Answer from the drawing. Dimensions are ordinates in mm from the lowest x, y and z of the part. A direction names the side the tool comes from. Coordinates: 2 decimals unless noted, no trailing zeros. Order: outer loops, then holes, each group sorted by start corner. A loop starts at its lowest first (then second) coordinate and runs counter-clockwise, first axis right, second up. Notation, with made-up numbers: (26.5, 61.25) -> (38.5, 61.25) arc R4 cw to (38.5, 68.25) -> close; hole circle Ø2 at (25.25, -2). An arc over 180 degrees is marked (long way). Answer as a JSON object with one key per item and string values. Group by question number.
1) A tool of negligible diameter and unlimited length cuts with its end or side. For the marked faces 1 and 2, from which of +Z, -Z, +X, -X, +Y, -Y can it reach the whole face along a straight path? Write none if from no direction.
2) Consider L1, parallel to Z at x = 33, y = 19.5; L2, parallel to X at y = 28, z = 31 (1 decimal); L3, parallel to X at y = 31.5, z = 26 (1 decimal). Determine where each line is inside the solid, lowest interval first.
3) Given pin 1 (4 mm diameter, centred on y = 19, z = 30, fed in from +X) (1 decimal); pin 2 (8 mm diameter, centred on y = 27.5, z = 22, fed in from -X); pin 3 (12 mm diameter, centred on y = 21, z = 25, fed in from +X), each flat-ended and moving along its own axis, determine where each tip first touches the part or whether it passes through.
4) Section B-B on x = 36 is taken. Determine the outline of the cut face in (y, z) (1 decimal), and give its area (3 significant figures).
5) Section C-C on z = 29 is taken. Determine the outline of the cut face in (x, y), and give its area (3 significant figures).
6) Section A-A on y = 30 is taken. Determine the outline of the cut face in (x, z).
7) Section D-D on x = 14 is taken. Determine the outline of the cut face in (y, z) (1 decimal), and give its area (3 significant figures).
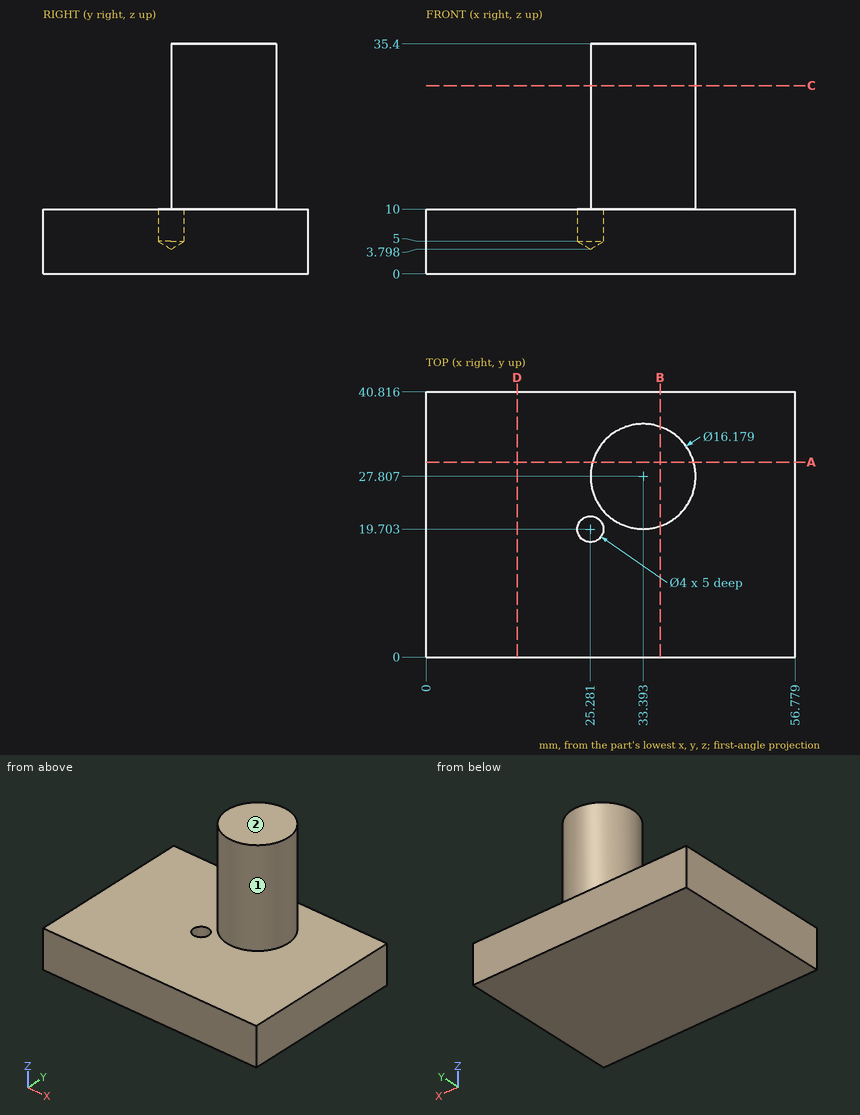
Worked answers:
{
 "1": {"face 1": "+Z", "face 2": "+Z, +X, -X, +Y, -Y"},
 "2": {"L1": "z = 0 to 10", "L2": "x = 25.3 to 41.5", "L3": "x = 26.2 to 40.6"},
 "3": {"pin 1": "stops at x = 37.8", "pin 2": "stops at x = 25.3", "pin 3": "stops at x = 41.44"},
 "4": {"outline": "(0, 0) -> (40.8, 0) -> (40.8, 10) -> (35.5, 10) -> (35.5, 35.4) -> (20.1, 35.4) -> (20.1, 10) -> (0, 10) -> close", "area": "797 mm²"},
 "5": {"outline": "circle Ø16.18 at (33.39, 27.81)", "area": "206 mm²"},
 "6": {"outline": "(0, 0) -> (56.78, 0) -> (56.78, 10) -> (41.18, 10) -> (41.18, 35.4) -> (25.61, 35.4) -> (25.61, 10) -> (0, 10) -> close"},
 "7": {"outline": "(0, 0) -> (40.8, 0) -> (40.8, 10) -> (0, 10) -> close", "area": "408 mm²"}
}
